Source: CAD feature listing. Evaluate the final solid. Frame: model axes, mm. Round coordinates to 2 decimals unless told otherwise and drop trailing zeros. Order: outer loops, then holes, each group sorted by start corner. A loop starts at its lowest first (then second) coordinate and runs counter-clockwise, first axis right, second up. Notation, with made-up numbers: (-16.5, -34.75) -> (6.5, -34.75) arc R22 cw to (6.5, -0.75) -> close; hole circle Ø8 at (-7.5, 83.5). An arc over 180 degrees is marked (long way). Answer as CSV lines item,"result".
from build123d import *

# Parameters (mm, degrees)
SKETCH1_R         = 1.55
SKETCH1_R_2       = 2.25
SKETCH1_R_3       = 13
MOTOR_PLATE_DEPTH = 3


with BuildPart() as part:
    # Sketch1 → Motor_Plate (new body)
    with BuildSketch(Plane(origin=(0, 0, 0), x_dir=(1, 0, 0), z_dir=(0, 1, 0))):
        with BuildLine():
            Line((25.5, -29), (25.5, 21))
            ThreePointArc((25.5, 21), (24.621320344, 23.121320344), (22.5, 24))
            Line((22.5, 24), (-22.5, 24))
            ThreePointArc((-22.5, 24), (-24.621320344, 23.121320344), (-25.5, 21))
            Line((-25.5, 21), (-25.5, -29))
            ThreePointArc((-25.5, -29), (-24.621320344, -31.121320344), (-22.5, -32))
            Line((-22.5, -32), (22.5, -32))
            ThreePointArc((22.5, -32), (24.621320344, -31.121320344), (25.5, -29))
        make_face()
        with Locations(Location((22.5, -21, 0), (0, 0, 270))):
            Circle(SKETCH1_R, mode=Mode.SUBTRACT)
        with Locations(Location((-22.5, -21, 0), (0, 0, 270))):
            Circle(SKETCH1_R, mode=Mode.SUBTRACT)
        with Locations(Location((0, -28, 0), (0, 0, 270))):
            Circle(SKETCH1_R_2, mode=Mode.SUBTRACT)
        with Locations(Location((0, 12, 0), (0, 0, 270))):
            Circle(SKETCH1_R_2, mode=Mode.SUBTRACT)
        with Locations(Location((-22.5, 21, 0), (0, 0, 270))):
            Circle(SKETCH1_R, mode=Mode.SUBTRACT)
        with Locations(Location((20, -8, 0), (0, 0, 270))):
            Circle(SKETCH1_R_2, mode=Mode.SUBTRACT)
        with Locations(Location((22.5, 21, 0), (0, 0, 270))):
            Circle(SKETCH1_R, mode=Mode.SUBTRACT)
        with Locations(Location((-20, -8, 0), (0, 0, 270))):
            Circle(SKETCH1_R_2, mode=Mode.SUBTRACT)
        with Locations(Location((0, -8, 0), (0, 0, 270))):
            Circle(SKETCH1_R_3, mode=Mode.SUBTRACT)
    extrude(amount=MOTOR_PLATE_DEPTH)


solid = part.part
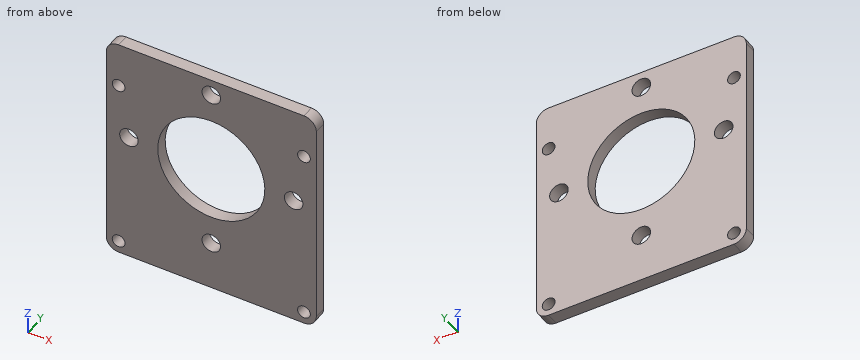
1. Line query: L1, parallel to X at y = 1.55, z = -21; L2, parallel to Z at x = -1, y = 1.8; L3, parallel to Z at x = 23, y = 0.7. Output: solid intervals per line, ascending. Write a range as [from, to].
Results below:
L1,"[-25.5, -24.05], [-20.95, 20.95], [24.05, 25.5]"
L2,"[-24, -14.02], [-9.98, -4.96], [20.96, 25.98], [30.02, 32]"
L3,"[-23.96, -22.47], [-19.53, 19.53], [22.47, 31.96]"
2. Section query C-C on x = -20. Return loops of the section in (y, z).
Results below:
outline,"(0, -24) -> (3, -24) -> (3, 5.75) -> (0, 5.75) -> close; (0, 10.25) -> (3, 10.25) -> (3, 32) -> (0, 32) -> close"
3. Pin query (flat end, axial travel): pin 1 (15.5 mm diameter, centred on x = 0, z = 8, fed in from -Y). Return the tip coordinate at first contact, or that it passes through.
Results below:
pin 1,"through"
4. Section query D-D on y = 2.15. Give the number of separate pieces and of enclosed holes in the cut face, and give its area (3 significant figures).
Results below:
separate pieces,"1"
enclosed holes,"9"
area,"2,220 mm2"
5. Section query A-A on x = 0. Return loops of the section in (y, z).
Results below:
outline,"(0, -24) -> (3, -24) -> (3, -14.25) -> (0, -14.25) -> close; (0, -9.75) -> (3, -9.75) -> (3, -5) -> (0, -5) -> close; (0, 21) -> (3, 21) -> (3, 25.75) -> (0, 25.75) -> close; (0, 30.25) -> (3, 30.25) -> (3, 32) -> (0, 32) -> close"
6. Section query B-B on z = -12. Return loops of the section in (x, y), and give its area (4 significant figures).
Results below:
outline,"(-25.5, 0) -> (-2.25, 0) -> (-2.25, 3) -> (-25.5, 3) -> close; (2.25, 0) -> (25.5, 0) -> (25.5, 3) -> (2.25, 3) -> close"
area,"139.5 mm2"
